The listing builds one solid part. Answer for the finished solid, in the listing's coordinates (mm). A direction names the side the tool comes from. Give positions to 0.01 mm unless a question says otherwise; leave off trailing zeros. Order: outer loops, then holes, each group sorted by start corner. A loop starts at its lowest first (then second) coordinate and runs counter-clockwise, first axis right, second up. Notation, with made-up numbers: (25.5, 29.5) - (55.5, 29.5) arc R19 ccw to (55.5, 51.5) - close; hole circle Ø8 at (-21.75, 78). An arc over 180 degrees is marked (long way). Use a Markdown table: item, result. Add a question column.
1) For faces 4 (the face through (-3.51, -5.01, 5.97)), 5 (the face through (-3.86, -5.01, -5.04)), 6 (the face through (-2.9, 2.1, -3.78)), determine the directions among +Z, -Z, +X, -X, +Y, -Y from which every point of the face is accessible in a straight line to the end or side of a thin tool.
2) Find section D-D, the plane z = -5.5. Determine the outline of the cut face in (x, y).
3) Find section B-B, the plane z = 0. Determine the outline of the cut face in (x, y), plus the area to 3 significant figures.
4) Straight lines are drawn through the part: line 1 (X direction, y = -4.25, z = 0); line 2 (Y direction, x = -3, z = 5.75); line 3 (Y direction, x = -0.5, z = -1.5). For each, find the intervals that lie inside material, in ascending order.
5) Find section C-C, the plane x = 5.75. Determine the outline of the cut face in (y, z), plus the area to 3 significant figures.
6) Flat-ended cylindrical pins translate along their axes: pin 1 (1.5 mm diameter, centred on x = -1.5, z = -1, fed in from -Y); pin 2 (3 mm diameter, centred on x = -2.5, y = -3.5, fed in from +Z). Find the tip coordinate at first contact, or state that the pin passes through.
7) Find section A-A, the plane y = -3.5. Determine the outline of the cut face in (x, z).
8) The mould has two halves that part along Z. Classify faces 1 (the face through (-5.593, 0.755, 2.909)), 2 (the face through (0, 5.08, 0)), 3 (the face through (0, 0, 0)): released by +Z, released by -Z, zero draft, split by the parting line, or undercut.
from build123d import *

# Parameters (mm, degrees)
SKETCH1_R           = 4.7625
BOSS_EXTRUDE1_DEPTH = 5.08
SKETCH1_4_R         = 6.35
BOSS_EXTRUDE4_DEPTH = 10.16
SKETCH7_R           = 6.304229739
BOSS_EXTRUDE5_DEPTH = 1.27
CHAMFER1_SIZE       = 2.126000066
CHAMFER1_SIZE2      = 1.60205596
SKETCH8_R           = 6.559510295
BOSS_EXTRUDE6_DEPTH = 0.254


with BuildPart() as part:
    # Sketch1 → Boss-Extrude1 (new body)
    with BuildSketch(Plane(origin=(0, 0, 0), x_dir=(1, 0, 0), z_dir=(0, 1, 0))):
        with Locations(Location((0, 0, 0), (0, 0, 270))):
            Circle(SKETCH1_R)
    extrude(amount=BOSS_EXTRUDE1_DEPTH)

    # Sketch7 → Boss-Extrude5 (add)
    with BuildSketch(Plane(origin=(0, 0, 0), x_dir=(1, 0, 0), z_dir=(0, 1, 0))):
        with Locations(Location((0, 0, 0), (0, 0, 270))):
            Circle(SKETCH7_R)
    extrude(amount=BOSS_EXTRUDE5_DEPTH)

    # Chamfer1
    chamfer1_edges = [part.edges().sort_by_distance(p)[0] for p in [
        (0, 5.08, -4.7625),
    ]]
    chamfer1_side = [part.faces().sort_by_distance(p)[0] for p in [
        (0, 3.175, -4.7625),
    ]]
    chamfer(chamfer1_edges, length=CHAMFER1_SIZE, length2=CHAMFER1_SIZE2, reference=chamfer1_side[0])



with BuildPart() as body_2:
    # Sketch1_4 → Boss-Extrude4 (new body)
    with BuildSketch(Plane(origin=(0, 0, 0), x_dir=(1, 0, 0), z_dir=(0, 1, 0))):
        Polygon((6.925488061, -3.998432396), (6.925488061, 3.998432396), (0, 7.996864793), (-6.925488061, 3.998432396), (-6.925488061, -3.998432396), (0, -7.996864793), align=None)
        with Locations(Location((0, 0, 0), (0, 0, 270))):
            Circle(SKETCH1_4_R, mode=Mode.SUBTRACT)
    extrude(amount=-BOSS_EXTRUDE4_DEPTH)


with BuildPart() as part_1:
    add(part.part)

    add(body_2.part)  # Boss-Extrude6 merges body 2
    # Sketch8 → Boss-Extrude6 (add)
    with BuildSketch(Plane(origin=(0, 0, 0), x_dir=(1, 0, 0), z_dir=(0, 1, 0))):
        with Locations(Location((0, 0, 0), (0, 0, 270))):
            Circle(SKETCH8_R)
    extrude(amount=BOSS_EXTRUDE6_DEPTH)


solid = part_1.part
The answers:
| question | item | result |
|---|---|---|
| 1 | face 4 | +Z, -X, +Y, -Y |
| 1 | face 5 | -Y |
| 1 | face 6 | +Y |
| 2 | outline | (-4.32, -10.16) - (-3.17, -10.16) - (-3.17, 0) - (3.17, 0) - (3.17, -10.16) - (4.32, -10.16) - (4.32, 0) - (3.57, 0) - (3.57, 0.25) - (3.08, 0.25) - (3.08, 1.27) - (-3.08, 1.27) - (-3.08, 0.25) - (-3.57, 0.25) - (-3.57, 0) - (-4.32, 0) - close |
| 3 | outline | (-6.93, -10.16) - (-6.35, -10.16) - (-6.35, 0) - (6.35, 0) - (6.35, -10.16) - (6.93, -10.16) - (6.93, 0) - (6.56, 0) - (6.56, 0.25) - (6.3, 0.25) - (6.3, 1.27) - (4.76, 1.27) - (4.76, 2.95) - (3.16, 5.08) - (-3.16, 5.08) - (-4.76, 2.95) - (-4.76, 1.27) - (-6.3, 1.27) - (-6.3, 0.25) - (-6.56, 0.25) - (-6.56, 0) - (-6.93, 0) - close |
| 3 | area | 60.7 mm2 |
| 4 | line 1 | -6.93 to -6.35, 6.35 to 6.93 |
| 4 | line 2 | -10.16 to 0.25 |
| 4 | line 3 | 0 to 5.08 |
| 5 | outline | (-10.16, -4.68) - (0, -4.68) - (0, -3.16) - (0.25, -3.16) - (0.25, -2.58) - (1.27, -2.58) - (1.27, 2.58) - (0.25, 2.58) - (0.25, 3.16) - (0, 3.16) - (0, 4.68) - (-10.16, 4.68) - (-10.16, 2.69) - (0, 2.69) - (0, -2.69) - (-10.16, -2.69) - close |
| 5 | area | 47.1 mm2 |
| 6 | pin 1 | y = 0 |
| 6 | pin 2 | z = 7.42 |
| 7 | outline | (-6.93, -4) - (0, -8) - (6.93, -4) - (6.93, 4) - (0, 8) - (-6.93, 4) - close; hole circle Ø12.7 at (0, 0) |
| 8 | face 1 | split by the parting line |
| 8 | face 2 | zero draft |
| 8 | face 3 | undercut |
